Geometry: final body of the model. Coordinates: model frame, mm. Give positions to 0.01 mm unless a question says otherwise; leave off trailing zeros. Order: outer loops, then holes, each group sorted by start corner. A loop starts at its lowest first (then second) coordinate and runs counter-clockwise, first axis right, second up. Notation, with made-up numbers: (-23, 25.5) -> (15, 25.5) arc R14 ccw to (15, 34.5) -> close; hole circle Ø6 at (-14, 10.25). An arc over 180 degrees is marked (long way). One line per question, with ' | ' between items.
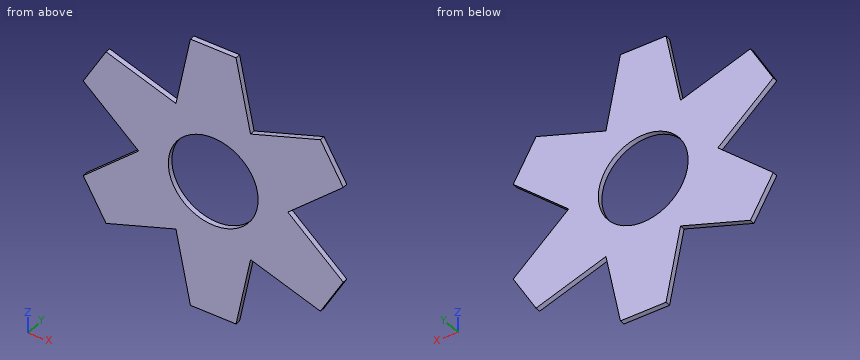
from build123d import *

# Parameters (mm, degrees)
F0_R     = 26.0720461281
F1_DEPTH = 3


with BuildPart() as f1:
    # F0 (on Front) → F1 (new body)
    with BuildSketch(Plane.XZ):
        Polygon((-13.25, 79.5), (-21.6506350946, 37.5), (0, 37.5), (0, 79.5), align=None)
        Polygon((0, 37.5), (-21.6506350946, 37.5), (-43.3012701892, 0), (-32.4759526419, -18.75), (-21.6506350946, -37.5), (0, -37.5), (21.6506350946, -37.5), (43.3012701892, 0), (21.6506350946, 37.5), align=None)
        Circle(F0_R, mode=Mode.SUBTRACT)
        Polygon((-43.3012701892, 0), (-21.6506350946, 37.5), (-62.2240208464, 51.2248376897), (-75.4740207353, 28.2751644252), align=None)
        Polygon((0, 79.5), (0, 37.5), (21.6506350946, 37.5), (13.25, 79.5), align=None)
        Polygon((-32.4759526419, -18.75), (-43.3012701892, 0), (-75.4740196009, -28.2751633999), (-68.8490196009, -39.75), align=None)
        Polygon((62.2240210561, 51.2248370699), (21.6506350946, 37.5), (43.3012701892, 0), (75.4740211672, 28.2751639337), align=None)
        Polygon((-21.6506350946, -37.5), (-32.4759526419, -18.75), (-68.8490196009, -39.75), (-62.2240196009, -51.2248366001), align=None)
        Polygon((75.4740211672, -28.2751639337), (43.3012701892, 0), (21.6506350946, -37.5), (62.2240210561, -51.2248370699), align=None)
        Polygon((0, -37.5), (-21.6506350946, -37.5), (-13.25, -79.5), (0, -79.5), align=None)
        Polygon((13.25, -79.5), (21.6506350946, -37.5), (0, -37.5), (0, -79.5), align=None)
    extrude(amount=F1_DEPTH)


solid = f1.part
1) Section B-B on y = -1.45. Return loops of the section in (x, z).
Check result:
outline: (-75.47, -28.28) -> (-62.22, -51.22) -> (-21.65, -37.5) -> (-13.25, -79.5) -> (13.25, -79.5) -> (21.65, -37.5) -> (62.22, -51.22) -> (75.47, -28.28) -> (43.3, 0) -> (75.47, 28.28) -> (62.22, 51.22) -> (21.65, 37.5) -> (13.25, 79.5) -> (-13.25, 79.5) -> (-21.65, 37.5) -> (-62.22, 51.22) -> (-75.47, 28.28) -> (-43.3, 0) -> close; hole circle Ø52.14 at (0, 0)
2) Section A-A on x = 0. Return loops of the section in (y, z).
Check result:
outline: (-3, -79.5) -> (0, -79.5) -> (0, -26.07) -> (-3, -26.07) -> close; (-3, 26.07) -> (0, 26.07) -> (0, 79.5) -> (-3, 79.5) -> close
3) Contact query for a flat-ended pin moving along its axis: pin 1 Ø1 at (x, y) = (-36.5, -2) entering from -Z. Output: stop coordinate, or through.
Check result:
pin 1: stops at z = -42.69
4) Material intervals for probe 1 along Z at (x, y) = (0, -1.6); probe 2 along X at (y, z) = (-2.1, 11); probe 3 along Z at (x, y) = (51.5, -2.05), sorted ascending. Write a range as from..to.
Check result:
probe 1: z = -79.5..-26.07, 26.07..79.5 | probe 2: x = -55.82..-23.64, 23.64..55.82 | probe 3: z = -47.6..-7.21, 7.21..47.6
5) Section D-D on x = -66. Return loops of the section in (y, z).
Check result:
outline: (-3, -44.68) -> (0, -44.68) -> (0, -19.95) -> (-3, -19.95) -> close; (-3, 19.95) -> (0, 19.95) -> (0, 44.68) -> (-3, 44.68) -> close
6) Section C-C on z = 46. Return loops of the section in (x, y).
Check result:
outline: (-65.24, -3) -> (-46.78, -3) -> (-46.78, 0) -> (-65.24, 0) -> close; (-19.95, -3) -> (19.95, -3) -> (19.95, 0) -> (-19.95, 0) -> close; (46.78, -3) -> (65.24, -3) -> (65.24, 0) -> (46.78, 0) -> close
